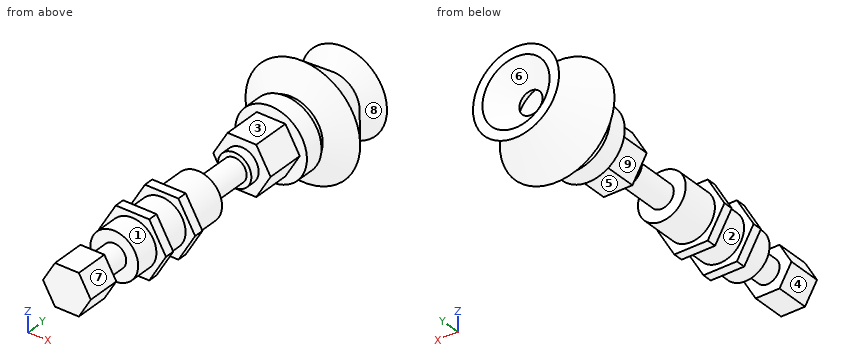
```python
from build123d import *

# Parameters (mm, degrees)
EXTRUDE_1_DEPTH = 7
SKETCH_2_R      = 2.5
EXTRUDE_2_DEPTH = 6
SKETCH_3_R      = 5
EXTRUDE_3_DEPTH = 23
EXTRUDE_4_DEPTH = 2
EXTRUDE_5_DEPTH = 2
SKETCH_6_R      = 2.5
EXTRUDE_6_DEPTH = 10
SKETCH_7_R      = 3.5
EXTRUDE_7_DEPTH = 2
EXTRUDE_8_DEPTH = 8
SKETCH_9_R      = 7.5
EXTRUDE_9_DEPTH = 4


with BuildPart() as part:
    # 草图1 → 凸台-拉伸1 (new body)
    with BuildSketch(Plane(origin=(0, 0, 0), x_dir=(1, 0, 0), z_dir=(0, 1, 0))):
        Polygon((-2.5, -4.330127019), (2.5, -4.330127019), (5, 0), (2.5, 4.330127019), (-2.5, 4.330127019), (-5, 0), align=None)
    extrude(amount=EXTRUDE_1_DEPTH)

    # 草图2 → 凸台-拉伸2 (add)
    with BuildSketch(Plane(origin=(0, 7, 0), x_dir=(1, 0, 0), z_dir=(0, 1, 0))):
        with Locations(Location((0, 0, 0), (0, 0, 270))):
            Circle(SKETCH_2_R)
    extrude(amount=EXTRUDE_2_DEPTH)

    # 草图3 → 凸台-拉伸3 (add)
    with BuildSketch(Plane(origin=(0, 13, 0), x_dir=(1, 0, 0), z_dir=(0, 1, 0))):
        with Locations(Location((0, 0, 0), (0, 0, 270))):
            Circle(SKETCH_3_R)
    extrude(amount=EXTRUDE_3_DEPTH)

    # 草图4 → 凸台-拉伸4 (add)
    with BuildSketch(Plane(origin=(0, 18, 0), x_dir=(-1, 0, 0), z_dir=(0, -1, 0))):
        Polygon((3.5, -6.062177826), (7, 0), (3.5, 6.062177826), (-3.5, 6.062177826), (-7, 0), (-3.5, -6.062177826), align=None)
    extrude(amount=-EXTRUDE_4_DEPTH)

    # 草图5 → 凸台-拉伸5 (add)
    with BuildSketch(Plane(origin=(0, 28, 0), x_dir=(1, 0, 0), z_dir=(0, 1, 0))):
        Polygon((-3.5, -6.062177826), (3.5, -6.062177826), (7, 0), (3.5, 6.062177826), (-3.5, 6.062177826), (-7, 0), align=None)
    extrude(amount=-EXTRUDE_5_DEPTH)

    # 草图6 → 凸台-拉伸6 (add)
    with BuildSketch(Plane(origin=(0, 36, 0), x_dir=(1, 0, 0), z_dir=(0, 1, 0))):
        with Locations(Location((0, 0, 0), (0, 0, 270))):
            Circle(SKETCH_6_R)
    extrude(amount=EXTRUDE_6_DEPTH)

    # 草图7 → 凸台-拉伸7 (add)
    with BuildSketch(Plane(origin=(0, 46, 0), x_dir=(1, 0, 0), z_dir=(0, 1, 0))):
        with Locations(Location((0, 0, 0), (0, 0, 270))):
            Circle(SKETCH_7_R)
    extrude(amount=EXTRUDE_7_DEPTH)

    # 草图8 → 凸台-拉伸8 (add)
    with BuildSketch(Plane(origin=(0, 48, 0), x_dir=(1, 0, 0), z_dir=(0, 1, 0))):
        Polygon((-3, 5.196152423), (-6, 0), (-3, -5.196152423), (3, -5.196152423), (6, 0), (3, 5.196152423), align=None)
    extrude(amount=EXTRUDE_8_DEPTH)

    # 草图9 → 凸台-拉伸9 (add)
    with BuildSketch(Plane(origin=(0, 56, 0), x_dir=(1, 0, 0), z_dir=(0, 1, 0))):
        with Locations(Location((0, 0, 0), (0, 0, 270))):
            Circle(SKETCH_9_R)
    extrude(amount=EXTRUDE_9_DEPTH)

    # 草图10 → 旋转2 (revolve)
    with BuildSketch(Plane(origin=(0, 0, 0), x_dir=(0, 0, -1), z_dir=(1, 0, 0)), mode=Mode.PRIVATE) as revolve_2_sk:
        Polygon((3.288999148, 64.305632713), (3.288999148, 60), (6.577998295, 60), (6.577998295, 61.5442992), (12, 64.711607127), (5.398859255, 73.199272663), (9, 76), (7.026755152, 76), (2.426170638, 71.892250876), (6.577998295, 67.242299418), align=None)
    revolve(revolve_2_sk.sketch.rotate(Axis((0, 76, 0), (0, -1, 0)), 180), axis=Axis((0, 76, 0), (0, -1, 0)))


solid = part.part
```
Source: CAD feature listing. Evaluate the final solid. Frame: model axes, mm. Face numbers are marked on the shaded views. A direction names the side the tool comes from. Give positions to 0.01 mm unless a question says otherwise; leave off trailing zeros. Write each loop counter-clockwise with the first axis right and the second up, starting at its lowest first coordinate (ties: lowest second). Pieces come first, ordered by that corner, then holes.
1. Pull-direction query (X, two-part tool) for the marked faces 6, 7, 8 and 9; classes: +X half, -X half, draft (parallel to the pull), parting line (faces both ways), or undercut.
2. First-contact query: pin 1 (5.5 mm diameter, centred on x = 0, z = 0, fed in from +Y); pin 2 (2 mm diameter, centred on x = 0.5, z = 0.5, fed in from +Y); pin 3 (6 mm diameter, centred on y = 27.5, z = -2.5, fed in from -X). Flat tips, straight axial feed; report the tip coordinate or a pass-through.
3. Section query A-A (y = 43). Return the cut outline in (x, z).
4. Material intervals for line 1 along X through (y, z) = (61.55, 0); line 2 along Y through (x, z) = (-5.25, 3.25); line 3 along Z through (x, y) = (-2.5, 5), sorted ascending.
5. Access query for the marked faces 1, 2, 3, 4 and 5. Directions: +Z, -Z, +X, -X, +Y, -Y. A direction counts if a zero-diameter tool reaches every point of the face in a straight line with its end or side. Return the directions, or none.
Output values:
1. face 6: undercut
1. face 7: +X half
1. face 8: parting line
1. face 9: -X half
2. pin 1: stops at y = 72.18
2. pin 2: stops at y = 60
2. pin 3: stops at x = -7
3. outline: circle Ø5 at (0, 0)
4. line 1: x = -6.59 to -3.29, 3.29 to 6.59
4. line 2: y = 56 to 66.88, 67.69 to 72.2, 73.8 to 75.24
4. line 3: z = -4.33 to 4.33
5. face 1: -Y
5. face 2: none
5. face 3: +Z, +X, -X
5. face 4: -Z, -X, -Y
5. face 5: -Z, +X, -X
